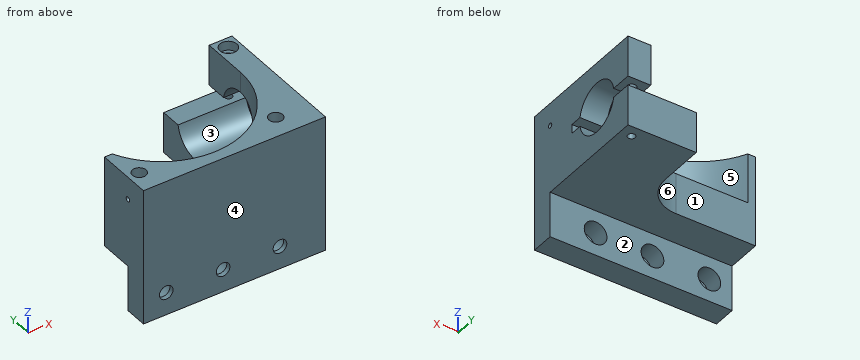
Autodesk Inventor part; units mm, degrees
ref_plane "YZ Plane" through (0, 0, 0) normal (1, 0, 0) x (0, 1, 0)
ref_plane "XZ Plane" through (0, 0, 0) normal (0, 1, 0) x (-1, 0, 0)
ref_plane "XY Plane" through (0, 0, 0) normal (0, 0, 1) x (1, 0, 0)
sketch "Sketch1" plane through (0, 0, 0) normal (0, 0, 1) x (1, 0, 0)
  line L0 (0, 32) -> (0, -52) construction
  line L1 (-59.4, 0) -> (76.4, 0) construction
  line L2 (-40, 20) -> (57, 20)
  line L3 (57, 20) -> (57, -40)
  line L4 (57, -40) -> (-40, -40)
  line L5 (-40, -40) -> (-40, 20)
  point P0 (0, 0)
  dimension "d0" = 20
  dimension "d1" = 40
  dimension "d2" = 40
  dimension "d3" = 57
extrude "Extrusion1" add sketch "Sketch1" against normal blind 40
sketch "Sketch2" plane through (0, 0, 0) normal (0, 0, 1) x (1, 0, 0)
  line L0 (-40, 20) -> (57, 20) construction
  line L1 (-40, -40) -> (-40, 20) construction
  line L2 (57, -40) -> (-40, -40) construction
  line L3 (57, 20) -> (57, -40) construction
  line L4 (0, 98) -> (0, -63) construction
  line L5 (-59.4, 0) -> (76.4, 0) construction
  line L6 (0, 40) -> (0, 0) construction
  line L7 (-40, 20) -> (57, 20)
  line L8 (-35, 40) -> (-35, 0)
  line L9 (35, 0) -> (35, 40)
  arc A0 (35, 40) -> (-35, 40) centre (0, 40) ccw
  arc A1 (-35, 0) -> (35, 0) centre (0, 0) ccw
  point P0 (0, 20)
  dimension "d6" = 70
extrude "Extrusion2" cut sketch "Sketch2" against normal blind 22
sketch "Sketch3" plane through (57, -40, 0) normal (1, 0, 0) x (0, 0, -1)
  line L0 (0, 60) -> (0, 0) construction
  line L1 (0, 0) -> (40, 0) construction
  line L2 (40, 60) -> (40, 0) construction
  line L3 (0, 60) -> (40, 60) construction
  line L4 (0, 40) -> (40, 40) construction
  line L5 (40, 0) -> (40, 60) construction
  line L6 (0, 60) -> (40, 60) construction
  line L7 (20, 60) -> (20, 0) construction
  circle A0 centre (20, 40) radius 11
  dimension "d9" = 22
extrude "Extrusion3" cut sketch "Sketch3" against normal blind 65
sketch "Sketch4" plane through (57, -40, 0) normal (1, 0, 0) x (0, 0, -1)
  circle A0 centre (20, 40) radius 11 construction
  line L0 (0, 60) -> (0, 0) construction
  line L1 (0, 0) -> (40, 0) construction
  line L2 (40, 60) -> (40, 0) construction
  line L3 (0, 60) -> (40, 60) construction
  line L4 (0, 60) -> (40, 60) construction
  line L5 (20, 60) -> (20, 0) construction
  line L6 (0, 0) -> (40, 0) construction
  line L7 (0, 40) -> (40, 40) construction
  line L8 (18, 60) -> (22, 60)
  line L9 (22, 60) -> (22, 24)
  line L10 (22, 24) -> (18, 24)
  line L11 (18, 24) -> (18, 60)
  dimension "d12" = 16
  dimension "d13" = 4
extrude "Extrusion4" cut sketch "Sketch4" against normal blind 70
sketch "Sketch6" plane through (0, 0, 0) normal (0, 0, 1) x (1, 0, 0)
  line L0 (0, 44) -> (0, -54) construction
  line L1 (-59.4, 0) -> (76.4, 0) construction
  line L2 (-30, 30) -> (30, 30) construction
  line L3 (30, 30) -> (30, -30) construction
  line L4 (30, -30) -> (-30, -30) construction
  line L5 (-30, -30) -> (-30, 30) construction
  point P0 (0, 0)
  dimension "d19" = 60
  dimension "d20" = 60
hole "Hole1" at (-30, -30, 0) at (30, -30, 0) direction (0, 0, -1) diameter 6 depth 30 tip angle 118
sketch "Sketch7" plane through (0, 0, -40) normal (0, 0, -1) x (-1, 0, 0)
  line L0 (40, 20) -> (-57, 20) construction
  line L1 (-57, 20) -> (-57, -40) construction
  line L2 (-57, -40) -> (40, -40) construction
  line L3 (40, -40) -> (40, 20) construction
  line L4 (0, -52) -> (0, 32) construction
  line L5 (-76.4, 0) -> (59.4, 0) construction
  line L6 (40, 20) -> (-15, 20)
  line L7 (-15, 20) -> (-15, -15)
  line L8 (-15, -15) -> (40, -15)
  line L9 (40, -15) -> (40, 20)
  point P0 (0, 0)
  dimension "d28" = 15
  dimension "d29" = 15
extrude "Extrusion6" cut sketch "Sketch7" against normal up to next
fillet "Fillet1" radius 15 1 edges at (15, -15, -31)
sketch "Sketch8" plane through (0, 0, -40) normal (0, 0, -1) x (-1, 0, 0)
  line L0 (40, -15) -> (0, -15) construction
  arc A0 (-15, 0) -> (0, -15) centre (0, 0) ccw construction
  line L1 (-15, 0) -> (-15, 20) construction
  line L2 (-15, 20) -> (-57, 20) construction
  line L3 (-57, 20) -> (-57, -40) construction
  line L4 (-57, -40) -> (40, -40) construction
  line L5 (40, -40) -> (40, -15) construction
  line L6 (-57, 20) -> (-57, -40)
  line L7 (40, -40) -> (-57, -40)
  line L8 (-57, -40) -> (-57, -30)
  line L9 (-57, -30) -> (40, -30)
  line L10 (40, -30) -> (40, -40)
  point P0 (0, 0)
  dimension "d33" = 10
extrude "Extrusion7" add sketch "Sketch8" along normal blind 20
sketch "Sketch13" plane through (-40, -30, -40) normal (0, 1, 0) x (1, 0, 0)
  line L0 (40, 32) -> (40, -52) construction
  line L1 (97, 0) -> (0, 0) construction
  line L2 (97, 0) -> (97, 20) construction
  line L3 (0, 20) -> (97, 20) construction
  line L4 (0, 0) -> (0, 20) construction
  line L5 (97, -40) -> (97, 20) construction
  line L6 (97, 10) -> (0, 10) construction
  point P0 (40, -40)
  point P1 (40, 10)
  point P2 (65, 10)
  point P3 (90, 10)
  point P4 (15, 10)
  dimension "d60" = 25
  dimension "d61" = 25
  dimension "d62" = 25
hole "Hole4" at (0, -30, -50) at (25, -30, -50) at (50, -30, -50) at (-25, -30, -50) direction (0, -1, 0) diameter 6 end through all counterbore diameter 10 counterbore depth 8
sketch "Sketch14" plane through (0, 0, 0) normal (0, 0, 1) x (1, 0, 0)
  line L0 (-31.6228, -15) -> (-40, -15) construction
  line L1 (-40, -40) -> (-40, -15) construction
  line L2 (57, -40) -> (-40, -40) construction
  line L3 (57, 20) -> (57, -40) construction
  line L4 (35, 20) -> (57, 20) construction
  line L5 (35, 20) -> (35, 0) construction
  arc A0 (-31.6228, -15) -> (35, 0) centre (0, 0) ccw construction
  circle A1 centre (30, -30) radius 3 construction
  circle A2 centre (-30, -30) radius 3 construction
  line L6 (57, 15) -> (35, 15) construction
  point P0 (40, 15)
  dimension "d70" = 5
  dimension "d106" = 5
hole "Hole5" at (40, 15, 0) direction (0, 0, -1) diameter 4 end up to surface counterbore diameter 7.5 counterbore depth 4
sketch "Sketch15" plane through (0, 0, -22) normal (0, 0, 1) x (1, 0, 0)
  circle A0 centre (40, 15) radius 2 construction
  point P0 (0, 0)
hole "Hole6" at (40, 15, -22) direction (0, 0, -1) diameter 3.242 end through all
sketch "Sketch16" plane through (-40, -40, 0) normal (-1, 0, 0) x (0, 0, 1)
  line L0 (0, 25) -> (-40, 25) construction
  line L1 (-40, 10) -> (-40, 25) construction
  line L2 (-40, 10) -> (-60, 10) construction
  line L3 (-60, 0) -> (-60, 10) construction
  line L4 (0, 0) -> (-60, 0) construction
  line L5 (0, 0) -> (0, 25) construction
  line L6 (0, 13) -> (0, 7) construction
  line L7 (-30, 7) -> (-30, 13) construction
  line L8 (-30, 10) -> (0, 10) construction
  point P0 (0, 40)
  point P1 (-10, 10)
  dimension "d86" = 10
hole "Hole7" at (-40, -30, -10) direction (1, 0, 0) diameter 2.156 depth 8.865 tip angle 118
sketch "Sketch18" plane through (-40, -40, 0) normal (-1, 0, 0) x (0, 0, 1)
  circle A0 centre (-10, 10) radius 1.078
  line L0 (0, 25) -> (-40, 25)
  line L1 (-40, 10) -> (-40, 25)
  line L2 (-40, 10) -> (-60, 10)
  line L3 (-60, 0) -> (-60, 10)
  line L4 (0, 0) -> (-60, 0)
  line L5 (0, 0) -> (0, 25)
  point P0 (0, 40)
extrude "Extrusion10" cut sketch "Sketch18" against normal blind 5
sketch "Sketch19" plane through (57, -40, 0) normal (1, 0, 0) x (0, 0, -1)
  line L0 (18, 50.8167) -> (18, 60)
  line L1 (0, 60) -> (18, 60)
  line L2 (0, 60) -> (0, 0)
  line L3 (0, 0) -> (60, 0)
  line L4 (60, 10) -> (60, 0)
  line L5 (40, 10) -> (60, 10)
  line L6 (40, 60) -> (40, 10)
  line L7 (22, 60) -> (40, 60)
  line L8 (22, 60) -> (22, 50.8167)
  arc A0 (22, 29.1833) -> (22, 50.8167) centre (20, 40) ccw
  line L9 (22, 29.1833) -> (22, 24)
  line L10 (22, 24) -> (18, 24)
  line L11 (18, 24) -> (18, 29.1833)
  arc A1 (18, 50.8167) -> (18, 29.1833) centre (20, 40) ccw
  point P0 (0, 40)
extrude "Extrusion11" cut sketch "Sketch19" against normal blind 12
sketch "Sketch20" plane through (45, -40, 0) normal (1, 0, 0) x (0, 0, -1)
  line L0 (18, 60) -> (18, 50.8167) construction
  line L1 (0, 60) -> (18, 60) construction
  line L2 (0, 0) -> (0, 60) construction
  line L3 (60, 0) -> (0, 0) construction
  line L4 (60, 10) -> (60, 0) construction
  line L5 (40, 10) -> (60, 10) construction
  line L6 (40, 60) -> (40, 10) construction
  line L7 (22, 60) -> (40, 60) construction
  line L8 (22, 50.8167) -> (22, 60) construction
  arc A0 (22, 29.1833) -> (22, 50.8167) centre (20, 40) ccw construction
  line L9 (22, 24) -> (22, 29.1833) construction
  line L10 (18, 24) -> (22, 24) construction
  line L11 (18, 29.1833) -> (18, 24) construction
  arc A1 (18, 50.8167) -> (18, 29.1833) centre (20, 40) ccw construction
  line L12 (0, 7) -> (0, 13) construction
  line L13 (30, 13) -> (30, 7) construction
  circle A2 centre (10, 10) radius 1.078 construction
  point P0 (0, 40)
hole "Hole9" at (45, -30, -10) direction (-1, 0, 0) diameter 2.156 depth 15 tip angle 118
properties part number "Galvomount-22mm-diameter-Thorlabs-Left"
Model file for the job. Use its own axes, mm. Face numbers are marked on the shaded views. A direction names the side the tool comes from. Give positions to 0.01 mm unless a question says otherwise; leave off trailing zeros. Loops run counter-clockwise (first coordinate to the right, second up) from the corner with the lowest first, then second, coordinate; pieces in that order, holes last. Notation, with made-up numbers: (-4, 76) -> (48, 76) arc R38 ccw to (48, 115) -> close; hole circle Ø7 at (36.25, 13). An arc over 180 degrees is marked (long way). Use a Markdown table: item, result. Add a question column.
(1) Slice it at B-B on z = -50. List the corners of the cut face in (x, y), and give its area (3 significant figures).
(2) Slice it at A-A on x = 40. List the corners of the cut face in (y, z), and give its area (3 significant figures).
(3) Drop flat-ended pins along their axis: pin 1 Ø6 at (x, z) = (-12.5, -46.5) entering from +Y; pin 2 Ø3 at (y, z) = (13, -30) entering from -X; pin 3 Ø9.5 at (x, z) = (0, -50) entering from +Y. Give the stop position or say it passes through.
(4) Wall check: line 1 along X through (y, z) = (-34, -50); line 2 along X through (y, z) = (-33, -46); line 3 along Z through (x, y) = (25, -32). Give the ranges that are in metal, low to high.
(5) Slice it at C-C on y = 15. List the corners of the cut face in (x, z), and give its area (3 significant figures).
(6) Mould opens along X. For the marked faces 4, 5 and 6 say: +X half, -X half, draft (parallel to the pull), parting line (faces both ways), or undercut.
(7) Tool access for the marked faces 1, 2 and 3: list every direction of +Z, -Z, +X, -X, +Y, -Y with a clear straight run to the whole face (end or side of a thin tool).
(8) Slice it at D-D on x = 23. List the corners of the cut face in (y, z).
Filled sheet:
| question | item | result |
|---|---|---|
| 1 | outline | (-35, -40) -> (-28, -40) -> (-28, -38) -> (-30, -38) -> (-30, -30) -> (-35, -30) -> close; (-22, -40) -> (-3, -40) -> (-3, -38) -> (-5, -38) -> (-5, -30) -> (-20, -30) -> (-20, -38) -> (-22, -38) -> close; (3, -40) -> (22, -40) -> (22, -38) -> (20, -38) -> (20, -30) -> (5, -30) -> (5, -38) -> (3, -38) -> close; (28, -40) -> (45, -40) -> (45, -30) -> (30, -30) -> (30, -38) -> (28, -38) -> close |
| 1 | area | 524 mm2 |
| 2 | outline | (-40, -60) -> (-30, -60) -> (-30, -40) -> (13.38, -40) -> (13.38, -22) -> (10.82, -22) arc R11 cw to (-10.82, -22) -> (-16, -22) -> (-16, -18) -> (-10.82, -18) arc R11 cw to (10.82, -18) -> (13, -18) -> (13, -4) -> (11.25, -4) -> (11.25, 0) -> (-40, 0) -> close; (16.62, -40) -> (20, -40) -> (20, -22) -> (16.62, -22) -> close; (17, -18) -> (20, -18) -> (20, 0) -> (18.75, 0) -> (18.75, -4) -> (17, -4) -> close; hole circle Ø2.16 at (-30, -10) |
| 2 | area | 2,020 mm2 |
| 3 | pin 1 | y = -30 |
| 3 | pin 2 | x = 15 |
| 3 | pin 3 | y = -38 |
| 4 | line 1 | -35 to -30, -20 to -5, 5 to 20, 30 to 45 |
| 4 | line 2 | -35 to -28, -22 to -3, 3 to 22, 28 to 45 |
| 4 | line 3 | -60 to -55, -45 to 0 |
| 5 | outline | (15, -40) -> (38.38, -40) -> (38.38, -22) -> (15, -22) -> close; (35, -18) -> (38, -18) -> (38, -4) -> (36.25, -4) -> (36.25, 0) -> (35, 0) -> close; (41.62, -40) -> (45, -40) -> (45, -22) -> (41.62, -22) -> close; (42, -18) -> (45, -18) -> (45, 0) -> (43.75, 0) -> (43.75, -4) -> (42, -4) -> close |
| 5 | area | 576 mm2 |
| 6 | face 4 | draft |
| 6 | face 5 | undercut |
| 6 | face 6 | -X half |
| 7 | face 1 | +Z, -Z, -X, +Y |
| 7 | face 2 | -Z, +X, -X, +Y |
| 7 | face 3 | +X, -X |
| 8 | outline | (-40, -60) -> (-30, -60) -> (-30, -54.58) -> (-38, -54.58) -> (-38, -52.24) -> (-40, -52.24) -> close; (-40, -47.76) -> (-38, -47.76) -> (-38, -45.42) -> (-30, -45.42) -> (-30, -40) -> (20, -40) -> (20, -22) -> (10.82, -22) arc R11 cw to (-10.82, -22) -> (-26.38, -22) -> (-26.38, 0) -> (-40, 0) -> close |
